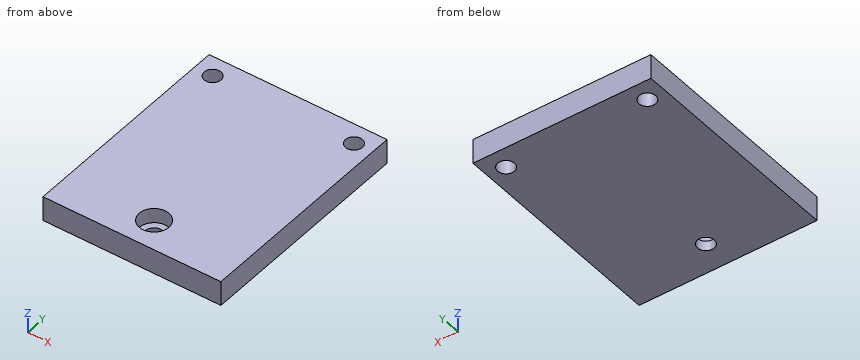
```python
from build123d import *

# Parameters (mm, degrees)
SKETCH025_R     = 1.7
PAD021_DEPTH    = 100
BOX_W           = 36
BOX_H           = 45
BOX_DEPTH       = 5
SKETCH026_R     = 3
POCKET002_DEPTH = 3


with BuildPart() as pad021:
    # Sketch025 → Pad021 (new body)
    with BuildSketch(Plane.XY.offset(-50)):
        with Locations((0, -19)):
            Circle(SKETCH025_R)
        with Locations((-14.3, 16)):
            Circle(SKETCH025_R)
        with Locations((14.3, 16)):
            Circle(SKETCH025_R)
    extrude(amount=PAD021_DEPTH)


with BuildPart() as pocket002:
    # Box → Box (new body)
    with BuildSketch(Plane(origin=(-18, -25, -12.4), x_dir=(1, 0, 0), z_dir=(0, 0, 1))):
        with Locations((18, 22.5)):
            Rectangle(BOX_W, BOX_H)
    extrude(amount=BOX_DEPTH)

    # Cut006: cut Pad021
    add(pad021.part, mode=Mode.SUBTRACT)

    # Sketch026 → Pocket002 (cut)
    with BuildSketch(Plane.XY.offset(-7.4)):
        with Locations((0, -19)):
            Circle(SKETCH026_R)
    extrude(amount=-POCKET002_DEPTH, mode=Mode.SUBTRACT)


solid = pocket002.part
```
Read the model definition and answer for the solid it produces. Units are mm, in the model's axes. Coordinates: 2 decimals unless noted, no trailing zeros. Write each loop counter-clockwise with the first axis right and the second up, starting at its lowest first coordinate (ties: lowest second). Pieces come first, ordered by that corner, then holes. Notation, with made-up numbers: (-23.75, -23.75) -> (22.25, -23.75) arc R24 cw to (22.25, 10.25) -> close; hole circle Ø4 at (-2, 88). An arc over 180 degrees is marked (long way). Answer as a JSON object with one key per item and string values.
Q1. The part is cut by section D-D on y = 16. Give the vertices of the cut face in (x, z), then the cut area to 3 significant figures.
The answers:
{"outline": "(-18, -12.4) -> (-16, -12.4) -> (-16, -7.4) -> (-18, -7.4) -> close; (-12.6, -12.4) -> (12.6, -12.4) -> (12.6, -7.4) -> (-12.6, -7.4) -> close; (16, -12.4) -> (18, -12.4) -> (18, -7.4) -> (16, -7.4) -> close", "area": "146 mm2"}
Q2. The part is cut by section C-C on y = -19. Give the vertices of the cut face in (x, z).
The answers:
{"outline": "(-18, -12.4) -> (-1.7, -12.4) -> (-1.7, -10.4) -> (-3, -10.4) -> (-3, -7.4) -> (-18, -7.4) -> close; (1.7, -12.4) -> (18, -12.4) -> (18, -7.4) -> (3, -7.4) -> (3, -10.4) -> (1.7, -10.4) -> close"}
Q3. Consider line 1 (X direction, y = 16, z = -9.45); line 2 (Y direction, x = 14.3, z = -8.6); line 3 (X direction, y = -19, z = -11.15). Determine where each line is inside the solid, lowest interval first. Write a range as [from, to].
The answers:
{"line 1": "x = [-18, -16], [-12.6, 12.6], [16, 18]", "line 2": "y = [-25, 14.3], [17.7, 20]", "line 3": "x = [-18, -1.7], [1.7, 18]"}
Q4. The part is cut by section B-B on x = 14.3. Give the vertices of the cut face in (y, z), then the cut area to 3 significant figures.
The answers:
{"outline": "(-25, -12.4) -> (14.3, -12.4) -> (14.3, -7.4) -> (-25, -7.4) -> close; (17.7, -12.4) -> (20, -12.4) -> (20, -7.4) -> (17.7, -7.4) -> close", "area": "208 mm2"}
Q5. The part is cut by section A-A on z = -8.25. Give the vertices of the cut face in (x, y).
The answers:
{"outline": "(-18, -25) -> (18, -25) -> (18, 20) -> (-18, 20) -> close; hole circle Ø3.4 at (-14.3, 16); hole circle Ø6 at (0, -19); hole circle Ø3.4 at (14.3, 16)"}
Q6. A flat-ended cylindrical pin translates along its axis: pin 1 Ø1.8 at (x, y) = (1, -20) entering from +Z. Find the tip coordinate at first contact, or state that the pin passes through.
The answers:
{"pin 1": "stops at z = -10.4"}
